```python
from build123d import *

# Parameters (mm, degrees)
F0_W     = 31.75
F0_H     = 6.35
F1_DEPTH = 12.7
F2_R     = 1.4204821808
F3_DEPTH = 1.27
F2_R_2   = 1.7458442661
F4_DEPTH = 0.508
F2_R_3   = 2.2844516469
F6_DEPTH = 12.7


# Not quite as in the source:
# - the program builds the solid bodies; features that only make, move or delete a surface that nothing else refers to are left out


with BuildPart() as f1:
    # F0 (on Front) → F1 (new body)
    with BuildSketch(Plane.XZ):
        with Locations((0, 15.875)):
            Rectangle(F0_W, F0_H)
        with Locations((0, 9.525)):
            Rectangle(F0_W, F0_H)
        with Locations((0, 3.175)):
            Rectangle(F0_W, F0_H)
        with Locations((0, -3.175)):
            Rectangle(F0_W, F0_H)
        with Locations((0, -9.525)):
            Rectangle(F0_W, F0_H)
        with Locations((0, -15.875)):
            Rectangle(F0_W, F0_H)
    extrude(amount=-F1_DEPTH)

    # F2 (on face) → F3 (join)
    with BuildSketch(Plane.XY.offset(19.05)):
        with Locations((-14.351, 6.35)):
            Circle(F2_R)
        with Locations((14.351, 6.35)):
            Circle(F2_R)
    extrude(amount=F3_DEPTH)

    # F2 (on face) → F4 (join)
    with BuildSketch(Plane.XY.offset(19.05)):
        with Locations((0, 6.35)):
            Circle(F2_R_2)
    extrude(amount=F4_DEPTH)

    # F2 (on face) → F6 (join)
    with BuildSketch(Plane.XY.offset(19.05)):
        with Locations((-9.271, 6.35)):
            Circle(F2_R_3)
        with Locations((9.271, 6.4142975025)):
            Circle(F2_R_3)
    extrude(amount=F6_DEPTH)


solid = f1.part
```
Input: part model. Units: mm. Frame: model coordinates. A direction names the side the tool comes from. Round coordinates to 2 decimals unless told otherwise and drop trailing zeros. Loops run counter-clockwise (first coordinate to the right, second up) from the corner with the lowest first, then second, coordinate; pieces in that order, holes last. Notation, with made-up numbers: (48.5, 18.25) -> (62.5, 18.25) arc R34 ccw to (62.5, 52.25) -> close; hole circle Ø2 at (-27, 75.25). An arc over 180 degrees is marked (long way). One line per item, written item: value.
(1) Pin query (flat end, axial travel): pin 1 (8 mm diameter, centred on x = -5.5, z = -0.5, fed in from -Y); pin 2 (4 mm diameter, centred on x = 0, y = 5.5, fed in from +Z); pin 3 (2 mm diameter, centred on x = 0, y = 3, fed in from +Z); pin 4 (3 mm diameter, centred on x = -15, y = 7, fed in from +Z). Return the tip coordinate at first contact, or that it passes through.
Geometry check:
pin 1: y = 0
pin 2: z = 19.56
pin 3: z = 19.05
pin 4: z = 20.32
(2) Section D-D (x = 10). Return the cut outline in (y, z).
Geometry check:
outline: (0, -19.05) -> (12.7, -19.05) -> (12.7, 19.05) -> (8.58, 19.05) -> (8.58, 31.75) -> (4.25, 31.75) -> (4.25, 19.05) -> (0, 19.05) -> close
(3) Material intervals for line 1 (Z direction, x = -10, y = 9.5); line 2 (Z direction, x = 0, y = 7); line 3 (X direction, y = 6, z = 27), sorted ascending. Write a range as [from, to].
Geometry check:
line 1: [-19.05, 19.05]
line 2: [-19.05, 19.56]
line 3: [-11.53, -7.01], [7.02, 11.52]
(4) Set-up query: faces 1 (the face through (-15.48, 5.49, 19.68)), 2 (the face through (14, 6, 20.32)), 3 (the face through (-14, 6, 20.32)), 4 (the face through (0, 6, 19.558)). Return all of +Z, -Z, +X, -X, +Y, -Y with unobstructed straight access to the full face (end or side cutting, diameter ignored); none if empty.
Geometry check:
face 1: +Z
face 2: +Z, +X, +Y, -Y
face 3: +Z, -X, +Y, -Y
face 4: +Z, +Y, -Y
(5) Section A-A (x = 0). Return the cut outline in (y, z).
Geometry check:
outline: (0, -19.05) -> (12.7, -19.05) -> (12.7, 19.05) -> (8.1, 19.05) -> (8.1, 19.56) -> (4.6, 19.56) -> (4.6, 19.05) -> (0, 19.05) -> close
(6) Section C-C (z = 24). Return the cut outline in (x, y).
Geometry check:
outline: circle Ø4.57 at (-9.27, 6.35); circle Ø4.57 at (9.27, 6.41)
(7) Section B-B (y = 9.25). Return the cut outline in (x, z) (3 decimals).
Geometry check:
outline: (-15.875, -19.05) -> (15.875, -19.05) -> (15.875, 19.05) -> (-15.875, 19.05) -> close
